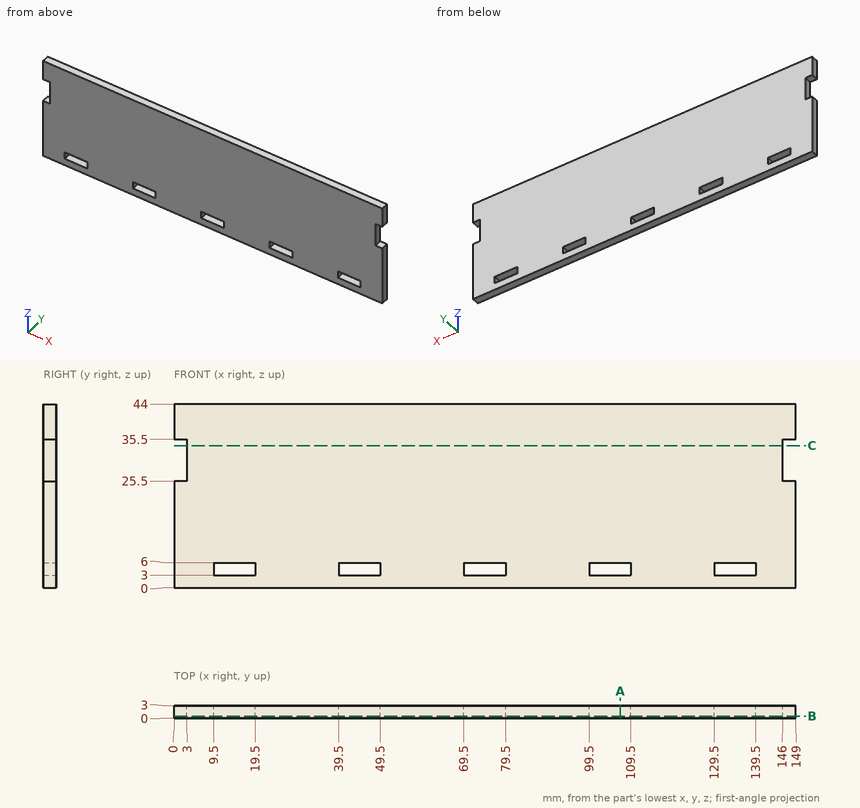
Job drawing, mm, ordinate dimensions from the low corner. One solid piece. Coordinates: 2 decimals unless noted, no trailing zeros. Loops run counter-clockwise (first coordinate to the right, second up) from the corner with the lowest first, then second, coordinate; pieces in that order, holes last. Notation, with made-up numbers: (20.25, 66) -> (58.25, 66) arc R25 ccw to (58.25, 104) -> close; hole circle Ø6 at (7.25, 33). An arc over 180 degrees is marked (long way). One line per item, written item: value.
1. Slice it at B-B on y = 0.45. Give the number of separate pieces and of enclosed holes in the cut face, and give its area (3 significant figures).
Answers:
separate pieces: 1
enclosed holes: 5
area: 6,350 mm^2
2. Slice it at A-A on x = 107. Write the cut outline in (y, z), and give its area (3 significant figures).
Answers:
outline: (0, 0) -> (3, 0) -> (3, 3) -> (0, 3) -> close; (0, 6) -> (3, 6) -> (3, 44) -> (0, 44) -> close
area: 123 mm^2
3. Drill centre lines: line 1 (Z direction, x = 139, y = 0.8); line 2 (X direction, y = 2.85, z = 30). Where is each one in solid material? Low to high. Write a range as [from, to].
Answers:
line 1: z = [0, 3], [6, 44]
line 2: x = [3, 146]
4. Slice it at C-C on z = 34. Write the cut outline in (x, y).
Answers:
outline: (3, 0) -> (146, 0) -> (146, 3) -> (3, 3) -> close
